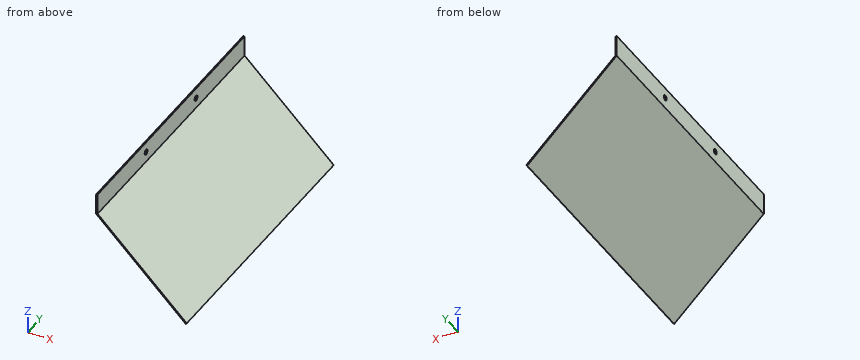
from build123d import *

# Parameters (mm, degrees)
BOSS_EXTRUDE1_DEPTH = 673.1
SKETCH2_R           = 6.35
CUT_EXTRUDE1_DEPTH  = 4.175


with BuildPart() as part:
    # Sketch1 → Boss-Extrude1 (new body)
    with BuildSketch(Plane(origin=(0, 0, 0), x_dir=(1, 0, 0), z_dir=(0, 1, 0))):
        Polygon((0, 0), (0, 50.8), (215.526146906, 266.326146906), (217.771210936, 264.081082875), (3.175, 49.484871939), (3.175, 0), align=None)
    extrude(amount=BOSS_EXTRUDE1_DEPTH)

    # Sketch2 → Cut-Extrude1 (cut, through all)
    with BuildSketch(Plane(origin=(3.175, 0, 0), x_dir=(0, 0, -1), z_dir=(1, 0, 0))):
        with Locations((24.74243597, 450.85)):
            Circle(SKETCH2_R)
        with Locations((24.74243597, 222.25)):
            Circle(SKETCH2_R)
    extrude(amount=-CUT_EXTRUDE1_DEPTH, mode=Mode.SUBTRACT)


solid = part.part
Model file for the job. Use its own axes, mm. Give positions to 0.01 mm unless a question says otherwise; leave off trailing zeros. Loops run counter-clockwise (first coordinate to the right, second up) from the corner with the lowest first, then second, coordinate; pieces in that order, holes last.
1) Flat gauge pins, fed straight in: pin 1 Ø1.5 at (x, y) = (190, 298.5) entering from +Z; pin 2 Ø6 at (y, z) = (337.5, -202.5) entering from +X; pin 3 Ø10 at (x, y) = (182, 542.5) entering from +Z. Where does each tip first touch, or does it go through?
2) Saw through at A-A (y = 222.25). Write the cut outline in (x, z) (3 decimals), plus the area to 3 significant figures.
3) Saw through at D-D (x = 67.5). Write the cut outline in (y, z).
4) Wall check: line 1 (X direction, y = 182.5, z = -23) (3 decimals); line 2 (X direction, y = 227, z = -67.5); line 3 (Z direction, x = 1, y = 450). Give the ranges that are in metal, low to high.
5) Saw through at C-C (z = -156). Write the cut outline in (x, y), plus the area to 3 significant figures.
6) Saw through at B-B (y = 294.5). Write the cut outline in (x, z) (3 decimals), plus the area to 3 significant figures.
Answer block:
1. pin 1: stops at z = -235.56
1. pin 2: stops at x = 159.19
1. pin 3: stops at z = -223.31
2. outline: (0, -50.8) - (215.526, -266.326) - (217.771, -264.081) - (3.175, -49.485) - (3.175, -31.092) - (0, -31.092) - close; (0, -18.392) - (3.175, -18.392) - (3.175, 0) - (0, 0) - close
2. area: 1,080 mm2
3. outline: (0, -118.3) - (673.1, -118.3) - (673.1, -113.81) - (0, -113.81) - close
4. line 1: x = 0 to 3.175
4. line 2: x = 16.7 to 21.19
4. line 3: z = -51.8 to -31.04, -18.45 to 0
5. outline: (105.2, 0) - (109.69, 0) - (109.69, 673.1) - (105.2, 673.1) - close
5. area: 3,020 mm2
6. outline: (0, -50.8) - (215.526, -266.326) - (217.771, -264.081) - (3.175, -49.485) - (3.175, 0) - (0, 0) - close
6. area: 1,120 mm2
